Geometry: final body of the model. Coordinates: model frame, mm. A direction names the side the tool comes from. Give positions to 0.01 mm unless a question says otherwise; leave off trailing zeros. Write each loop counter-clockwise with the first axis right and the second up, starting at its lowest first coordinate (ties: lowest second). Pieces come first, ordered by that corner, then holes. Notation, with made-up numbers: (65.5, -28.5) -> (117.5, -28.5) arc R18 ccw to (117.5, 3.5) -> close; hole circle Ø5 at (28, 16.25). An arc over 180 degrees is marked (long way). Answer in a Markdown table with one row per item. Add a question column.
Item 1: Access query for faces 3 (the cylindrical face through (25.154, -0.651, 58.957)), 4 (the flat face through (25, 42.5, 1)). Directions: +Z, -Z, +X, -X, +Y, -Y. A direction counts if a zero-diameter tool reaches every point of the face in a straight line with its end or side. Return the directions, or none.
Item 2: Section query C-C on y = 29. Output: boundary loops of the cut face in (x, z).
Item 3: First-contact query: P1, Ø17.5, axis at x = 26, y = -4.5, coming from the +Z side; P2, Ø2, axis at x = 12.5, y = 12, coming from the +Z side; P3, Ø24, axis at x = 54.5, y = 2.5, coming from the +Z side; P4, Ø6, axis at x = 28.5, y = 6.5, coming from the +Z side. Flat tips, straight axial feed; report the tip coordinate or a pass-through.
Item 4: Section query A-A on z = 9. Output: boundary loops of the cut face in (x, y).
Item 5: Section query D-D on z = 54. Output: boundary loops of the cut face in (x, y), plus the area to 3 significant figures.
Item 6: Material intervals for probe 1 along X at (y, z) = (-1, 28.5); probe 2 along Z at (x, y) = (2.5, 0); probe 3 along Z at (x, y) = (-1.5, -34), sorted ascending. Write a range as from..to.
Item 7: Draft query along X for faces 1 (the flat face through (-11, -1, 25)), 2 (the flat face through (24, 1, 0)). Return one class per face: +X half, -X half, draft (parallel to the pull), parting line (faces both ways), or undercut.
Item 8: Section query B-B on x = -2.5. Output: boundary loops of the cut face in (y, z), plus the area to 3 significant figures.
Autodesk Fusion 360 part; units mm, degrees
sketch "Sketch1" plane through (0, 0, 0) normal (0, 0, 1) x (1, 0, 0)
  line L0 (11, -40) -> (-11, -40)
  line L1 (-11, -42.5) -> (-11, 42.5)
  line L2 (-11, 40) -> (11, 40)
  line L3 (11, 42.5) -> (11, -42.5)
  line L4 (-13.5, -42.5) -> (-13.5, 42.5)
  line L5 (-13.5, 42.5) -> (13.5, 42.5)
  line L6 (13.5, 42.5) -> (13.5, -42.5)
  line L7 (13.5, -42.5) -> (-13.5, -42.5)
  dimension "d1" = 22
  dimension "d2" = 80
extrude "Extrude1" add sketch "Sketch1" along normal blind 3 makes body 1
extrude "Extrude2" add sketch "Sketch1" along normal blind 60 contours L3 L5 L6 L7 | L1 L4 L5 L7 bodies 1
fillet "Fillet1" radius 42.5 4 edges at (12.25, -42.5, 60) (-12.25, -42.5, 60) (12.25, 42.5, 60) (-12.25, 42.5, 60) on bodies 1
sketch "Sketch2" plane through (13.5, 0, 0) normal (1, 0, 0) x (0, 1, 0)
  arc A0 (42.5, 17.5) -> (-42.5, 17.5) centre (0, 17.5) ccw
  line L0 (-42.5, 17.5) -> (-42.5, 0)
  line L1 (-42.5, 0) -> (42.5, 0)
  line L2 (42.5, 0) -> (42.5, 17.5)
  circle A1 centre (0, 54) radius 5
  dimension "d10" = 10
extrude "Extrude3" add sketch "Sketch2" against normal blind 27 contours A1 bodies 1
pattern_linear "R-Pattern1" count 3 spacing 25 along (1, 0, 0) of bodies 1 makes body 2 at (38.5, 0.0028, 31.6723) makes body 3 at (63.5, 0.0028, 31.6723)
combine "Combine1" operation add target body 1 tool bodies 2 3
Findings below:
| question | item | result |
|---|---|---|
| 1 | face 3 | none |
| 1 | face 4 | +Z, -Z, +X, -X, +Y |
| 2 | outline | (-13.5, 0) -> (63.5, 0) -> (63.5, 48.57) -> (61, 48.57) -> (61, 3) -> (39, 3) -> (39, 48.57) -> (36, 48.57) -> (36, 3) -> (14, 3) -> (14, 48.57) -> (11, 48.57) -> (11, 3) -> (-11, 3) -> (-11, 48.57) -> (-13.5, 48.57) -> close |
| 3 | P1 | stops at z = 59 |
| 3 | P2 | stops at z = 58.55 |
| 3 | P3 | stops at z = 60 |
| 3 | P4 | stops at z = 57.57 |
| 4 | outline | (-13.5, -42.5) -> (-11, -42.5) -> (-11, 42.5) -> (-13.5, 42.5) -> close; (11, -42.5) -> (14, -42.5) -> (14, 42.5) -> (11, 42.5) -> close; (36, -42.5) -> (39, -42.5) -> (39, 42.5) -> (36, 42.5) -> close; (61, -42.5) -> (63.5, -42.5) -> (63.5, 42.5) -> (61, 42.5) -> close |
| 5 | outline | (-13.5, -21.78) -> (-11, -21.78) -> (-11, -5) -> (11, -5) -> (11, -21.78) -> (14, -21.78) -> (14, -5) -> (36, -5) -> (36, -21.78) -> (39, -21.78) -> (39, -5) -> (61, -5) -> (61, -21.78) -> (63.5, -21.78) -> (63.5, 21.78) -> (61, 21.78) -> (61, 5) -> (39, 5) -> (39, 21.78) -> (36, 21.78) -> (36, 5) -> (14, 5) -> (14, 21.78) -> (11, 21.78) -> (11, 5) -> (-11, 5) -> (-11, 21.78) -> (-13.5, 21.78) -> close |
| 5 | area | 1,140 mm^2 |
| 6 | probe 1 | x = -13.5..-11, 11..14, 36..39, 61..63.5 |
| 6 | probe 2 | z = 0..3, 49..59 |
| 6 | probe 3 | z = 0..3 |
| 7 | face 1 | undercut |
| 7 | face 2 | draft |
| 8 | outline | (-42.5, 0) -> (42.5, 0) -> (42.5, 3) -> (-42.5, 3) -> close; circle Ø10 at (0, 54) |
| 8 | area | 334 mm^2 |
